Check sheet for the modelled part. Datum: model origin and axes. Units: mm. A direction names the side the tool comes from. Round coordinates to 2 decimals unless told otherwise and drop trailing zeros. Write each loop counter-clockwise with the first axis right and the second up, starting at its lowest first coordinate (ties: lowest second). Pieces come first, ordered by that corner, then holes. Notation, with made-up numbers: M 50.5,3.5 L 64.5,3.5 A19 cw 64.5,31.5 Z; hole C 50.5,64 d6. An arc over 180 degrees is marked long. Put each result on its own line as item: value.
```python
from build123d import *

# Parameters (mm, degrees)
F0_W     = 184.15
F0_H     = 38.1
F1_DEPTH = 939.8
F3_DEPTH = 38.1
F4_R     = 6.35
F5_DEPTH = 38.101


# Not quite as in the source:
# - a feature names something its author has since deleted; it is built from what else it names


with BuildPart() as f1:
    # F0 (on Right) → F1 (new body)
    with BuildSketch(Plane.YZ):
        with Locations((1.8085447712, 0)):
            Rectangle(F0_W, F0_H)
    extrude(amount=F1_DEPTH)

    # F2 (on face) → F3 (cut)
    with BuildSketch(Plane.XZ.offset(90.2664552288)):
        with BuildLine():
            Line((117.475, 9.525), (60.325, 9.525))
            ThreePointArc((60.325, 9.525), (50.8, 0), (60.325, -9.525))
            Line((60.325, -9.525), (117.475, -9.525))
            ThreePointArc((117.475, -9.525), (127, 0), (117.475, 9.525))
        make_face()
        with BuildLine():
            Line((307.975, 9.525), (250.825, 9.525))
            ThreePointArc((250.825, 9.525), (241.3, 0), (250.825, -9.525))
            Line((250.825, -9.525), (307.975, -9.525))
            ThreePointArc((307.975, -9.525), (317.5, 0), (307.975, 9.525))
        make_face()
        with BuildLine():
            Line((688.975, 9.525), (631.825, 9.525))
            ThreePointArc((631.825, 9.525), (622.3, 0), (631.825, -9.525))
            Line((631.825, -9.525), (688.975, -9.525))
            ThreePointArc((688.975, -9.525), (698.5, 0), (688.975, 9.525))
        make_face()
        with BuildLine():
            Line((879.475, 9.525), (822.325, 9.525))
            ThreePointArc((822.325, 9.525), (812.8, 0), (822.325, -9.525))
            Line((822.325, -9.525), (879.475, -9.525))
            ThreePointArc((879.475, -9.525), (889, 0), (879.475, 9.525))
        make_face()
        with BuildLine():
            Line((485.775, 9.525), (454.025, 9.525))
            ThreePointArc((454.025, 9.525), (444.5, 0), (454.025, -9.525))
            Line((454.025, -9.525), (485.775, -9.525))
            ThreePointArc((485.775, -9.525), (495.3, 0), (485.775, 9.525))
        make_face()
    extrude(amount=-F3_DEPTH, mode=Mode.SUBTRACT)

    # F4 (on face) → F5 (cut, through all)
    with BuildSketch(Plane.XY.offset(19.05)):
        with Locations((88.9, -71.2164552288)):
            Circle(F4_R)
        with Locations((279.4, -71.2164552288)):
            Circle(F4_R)
        with Locations((469.9, -71.2164552288)):
            Circle(F4_R)
        with Locations((660.4, -71.2164552288)):
            Circle(F4_R)
        with Locations((850.9, -71.2164552288)):
            Circle(F4_R)
    extrude(amount=-F5_DEPTH, mode=Mode.SUBTRACT)


solid = f1.part
```
1. Scan lines: probe 1 along Y at (x, z) = (850, -16); probe 2 along X at (y, z) = (-68, -8); probe 3 along Y at (x, z) = (469.9, -13.75). Record each from-to range of solid material in increasing order.
Computed values:
probe 1: y = -90.27 to -77.5, -64.93 to 93.88
probe 2: x = 0 to 55.16, 122.64 to 245.66, 313.14 to 448.86, 490.94 to 626.66, 694.14 to 817.16, 884.64 to 939.8
probe 3: y = -90.27 to -77.57, -64.87 to 93.88
2. Cross-section at A-A (z = 0). Enter the section's corners in (x, y), then the cut area to 3 significant figures.
Computed values:
outline: M 0,-90.27 L 50.8,-90.27 L 50.8,-52.17 L 127,-52.17 L 127,-90.27 L 241.3,-90.27 L 241.3,-52.17 L 317.5,-52.17 L 317.5,-90.27 L 444.5,-90.27 L 444.5,-52.17 L 495.3,-52.17 L 495.3,-90.27 L 622.3,-90.27 L 622.3,-52.17 L 698.5,-52.17 L 698.5,-90.27 L 812.8,-90.27 L 812.8,-52.17 L 889,-52.17 L 889,-90.27 L 939.8,-90.27 L 939.8,93.88 L 0,93.88 Z
area: 160,000 mm2
3. Access from +Z, -Z, +X, -X, +Y, -Y to the whole of each face (thin tool, end or side, straight path). Record for faces 1 (the flat face through (477, -71, 9.525)), 2 (the flat face through (463, -90.266, -13)).
Computed values:
face 1: -Y
face 2: +Z, -Z, +X, -X, -Y
4. Release check for a two-part mould opening along X. For faces 3 (the flat face through (463, 1, -19.05)), 4 (the flat face through (279, -52.166, 0)) record: +X half, -X half, draft (parallel to the pull), parting line (faces both ways), or undercut.
Computed values:
face 3: draft
face 4: undercut
5. Depth check by flat-ended pin: pin 1 Ø7.5 at (x, y) = (279.4, -71.22) entering from +Z. Enter the tip coordinate at first touch or a pass-through.
Computed values:
pin 1: passes through
